Check sheet for the modelled part. Datum: model origin and axes. Units: mm. A direction names the side the tool comes from. Give positions to 0.01 mm unless a question says otherwise; leave off trailing zeros. Write each loop counter-clockwise with the first axis right and the second up, starting at its lowest first coordinate (ties: lowest second). Pieces come first, ordered by that corner, then holes. Notation, with made-up numbers: (32, 80.5) -> (89, 80.5) arc R30 ccw to (89, 107.5) -> close; hole circle Ø11 at (-17, 6). An arc over 180 degrees is marked (long way). Write each question's results on one line, items separated by ' | '. Start each with the question number.
```python
from build123d import *

# Parameters (mm, degrees)
BOSS_EXTRUDE1_DEPTH = 15
SKETCH5_R           = 15
CUT_EXTRUDE1_DEPTH  = 31


with BuildPart() as part:
    # Sketch4 → Boss-Extrude1 (new body)
    with BuildSketch(Plane(origin=(0, 0, 0), x_dir=(1, 0, 0), z_dir=(0, 1, 0))):
        with BuildLine():
            Line((0, -50), (200, -50))
            ThreePointArc((200, -50), (233.424270678, -67.095996649), (239.124306246, -104.203469835))
            Line((239.124306246, -104.203469835), (289.124306246, -104.203469835))
            ThreePointArc((289.124306246, -104.203469835), (268.559290197, -31.577195792), (200, 0))
            Line((200, 0), (0, 0))
            Line((0, 0), (0, -50))
        make_face()
    extrude(amount=BOSS_EXTRUDE1_DEPTH)

    # Sketch5 → Cut-Extrude1 (cut)
    with BuildSketch(Plane(origin=(0, 15, 0), x_dir=(1, 0, 0), z_dir=(0, 1, 0))):
        with Locations(Location((264.124306246, -79.466665475, 0), (0, 0, 270))):
            Circle(SKETCH5_R)
    extrude(amount=-CUT_EXTRUDE1_DEPTH, mode=Mode.SUBTRACT)


solid = part.part
```
Item 1: Depth check by flat-ended pin: pin 1 Ø5 at (y, z) = (3, 93.5) entering from -X; pin 2 Ø1.5 at (x, y) = (143, 4) entering from +Z; pin 3 Ø2 at (y, z) = (4.5, 35.5) entering from +X. Enter the tip coordinate at first touch or a pass-through.
Item 2: Mould release check, pull along Z, two halves, no side actions. Record for faces 3 (the flat face through (143, 0, 28)), 4 (the flat face through (101, 7, 0)), 5 (the cylindrical face through (233.102, 7.395, 66.656)): pulls with the +Z half, pulls with the -Z half, needs draft (parallel to the pull), parting line crosses it, or undercut.
Item 3: Section check C-C on z = 42. Record the boundary of the cut face in (x, y).
Item 4: Set-up check for faces 1 (the flat face through (99, 7, 50)), 2 (the cylindrical face through (255, 7.6, 67.56)): record each of +Z, -Z, +X, -X, +Y, -Y from which the full face is reachable in a straight line by a thin tool's end or side.
Item 5: Section check A-A on y = 9.75. Record the boundary of the cut face in (x, z), then the cut area to 3 significant figures.
Item 6: Section check B-B on x = 102. Record the boundary of the cut face in (y, z), then the cut area to 3 significant figures.
Item 7: Thickness scan on probe 1 along Z at (x, y) = (102.5, 4.5); probe 2 along X at (y, z) = (11.25, 88); probe 3 along X at (y, z) = (11.5, 10). Record the ranges inside material, lowest first. Write a range as from..to.
Check sheet entries:
1) pin 1: stops at x = 240.94 | pin 2: stops at z = 50 | pin 3: stops at x = 272.48
2) face 3: needs draft | face 4: pulls with the -Z half | face 5: undercut
3) outline: (0, 0) -> (276.25, 0) -> (276.25, 15) -> (0, 15) -> close
4) face 1: +Z, -X, +Y, -Y | face 2: +Y, -Y
5) outline: (0, 0) -> (200, 0) arc R90.22 ccw to (289.12, 104.2) -> (239.12, 104.2) arc R41.22 cw to (200, 50) -> (0, 50) -> close; hole circle Ø30 at (264.12, 79.47) | area: 15,100 mm^2
6) outline: (0, 0) -> (15, 0) -> (15, 50) -> (0, 50) -> close | area: 750 mm^2
7) probe 1: z = 0..50 | probe 2: x = 241.1..251.79, 276.46..290.19 | probe 3: x = 0..241.28
